from build123d import *

# Parameters (mm, degrees)
SKETCH1_W           = 55
SKETCH1_H           = 36
SKETCH1_R           = 2
BOSS_EXTRUDE1_DEPTH = 10
SKETCH2_W           = 7
SKETCH2_H           = 20
SKETCH2_H_2         = 17.5
BOSS_EXTRUDE2_DEPTH = 21
SKETCH3_R           = 1.25
CUT_EXTRUDE1_DEPTH  = 10
CUT_EXTRUDE2_DEPTH  = 5.5
LPATTERN1_COUNT     = 2
LPATTERN1_PITCH     = 28
FILLET1_R           = 1


with BuildPart() as part:
    # Sketch1 → Boss-Extrude1 (new body)
    with BuildSketch(Plane.XY):
        with Locations((27.5, -18)):
            Rectangle(SKETCH1_W, SKETCH1_H)
        with Locations((13.5, -4.5)):
            Circle(SKETCH1_R, mode=Mode.SUBTRACT)
        with Locations((41.5, -4.5)):
            Circle(SKETCH1_R, mode=Mode.SUBTRACT)
    extrude(amount=BOSS_EXTRUDE1_DEPTH)

    # Sketch2 → Boss-Extrude2 (add)
    with BuildSketch(Plane.XZ.offset(36)):
        with Locations((3.5, 20)):
            Rectangle(SKETCH2_W, SKETCH2_H)
        with Locations((51.5, 18.75)):
            Rectangle(SKETCH2_W, SKETCH2_H_2)
    extrude(amount=-BOSS_EXTRUDE2_DEPTH)

    # Sketch3 → Cut-Extrude1 (cut)
    with BuildSketch(Plane(origin=(0, -15, 0), x_dir=(1, 0, 0), z_dir=(0, 1, 0))):
        with Locations(Location((3.5, -15, 0), (0, 0, 270))):
            Circle(SKETCH3_R)
        with Locations(Location((51.5, -15, 0), (0, 0, 270))):
            Circle(SKETCH3_R)
        with Locations(Location((51.5, -25, 0), (0, 0, 270))):
            Circle(SKETCH3_R)
        with Locations(Location((3.5, -25, 0), (0, 0, 270))):
            Circle(SKETCH3_R)
    extrude(amount=-CUT_EXTRUDE1_DEPTH, mode=Mode.SUBTRACT)

    # Sketch4 → Cut-Extrude2 (cut)
    with BuildSketch(Plane.XY.offset(10)):
        Polygon((11.91228676, -1.75), (10.324573519, -4.5), (11.91228676, -7.25), (15.08771324, -7.25), (16.675426481, -4.5), (15.08771324, -1.75), align=None)
    cut_extrude2 = extrude(amount=-CUT_EXTRUDE2_DEPTH, mode=Mode.SUBTRACT)

    # LPattern1: Cut-Extrude2 ×2
    with Locations(*[(i * LPATTERN1_PITCH, 0, 0) for i in range(1, LPATTERN1_COUNT)]):
        add(cut_extrude2, mode=Mode.SUBTRACT)

    # Fillet1
    fillet1_edges = [part.edges().sort_by_distance(p)[0] for p in [
        (0, -25.5, 30),
        (7, -25.5, 30),
        (7, -25.5, 10),
        (55, -25.5, 27.5),
        (48, -25.5, 10),
        (48, -25.5, 27.5),
    ]]
    fillet(fillet1_edges, radius=FILLET1_R)


solid = part.part
Work out the finished part from the listing and answer in its coordinate system (mm). A direction names the side the tool comes from. Give positions to 0.01 mm unless a question says otherwise; leave off trailing zeros. Loops run counter-clockwise (first coordinate to the right, second up) from the corner with the lowest first, then second, coordinate; pieces in that order, holes last. Notation, with made-up numbers: (30.5, 54) - (42.5, 54) arc R21 cw to (42.5, 84) - close; hole circle Ø4 at (78, 18). An arc over 180 degrees is marked (long way). Answer in a Markdown table with one row per item.
(1) Section C-C (z = 12.75) is taken. Give the vertices of the cut face in (x, y), and give its area (3 significant figures).
Results list:
| item | result |
|---|---|
| outline | (0, -36) - (7, -36) - (7, -15) - (0, -15) - close; (48, -36) - (55, -36) - (55, -15) - (48, -15) - close |
| area | 294 mm² |
(2) Section A-A (x = 13.5) is taken. Give the vertices of the cut face in (y, z), and give its area (3 significant figures).
Results list:
| item | result |
|---|---|
| outline | (-36, 0) - (-6.5, 0) - (-6.5, 4.5) - (-7.25, 4.5) - (-7.25, 10) - (-36, 10) - close; (-2.5, 0) - (0, 0) - (0, 10) - (-1.75, 10) - (-1.75, 4.5) - (-2.5, 4.5) - close |
| area | 312 mm² |
(3) Section B-B (y = -19) is taken. Give the vertices of the cut face in (x, z).
Results list:
| item | result |
|---|---|
| outline | (0, 0) - (55, 0) - (55, 26.5) arc R1 ccw to (54, 27.5) - (49, 27.5) arc R1 ccw to (48, 26.5) - (48, 11) arc R1 cw to (47, 10) - (8, 10) arc R1 cw to (7, 11) - (7, 29) arc R1 ccw to (6, 30) - (1, 30) arc R1 ccw to (0, 29) - close; hole circle Ø2.5 at (3.5, 15); hole circle Ø2.5 at (3.5, 25); hole circle Ø2.5 at (51.5, 15); hole circle Ø2.5 at (51.5, 25) |
(4) For a pull along X with two mould halves and no side action, classify faces 6 (the face through (2.74, -19.93, 14.01)), 7 (the face through (27, -36, 9)) as pulls with the +X half, pulls with the -X half, needs draft (parallel to the pull), parting line crosses it, or undercut.
Results list:
| item | result |
|---|---|
| face 6 | undercut |
| face 7 | needs draft |
(5) Consider L1, parallel to X at y = -19, z = 15; L2, parallel to X at y = -4.5, z = 2.3; L3, parallel to Y at x = 14, z = 9. Determine where each line is inside the solid, lowest interval first. Write a range as [from, to].
Results list:
| item | result |
|---|---|
| L1 | x = [0, 2.25], [4.75, 7], [48, 50.25], [52.75, 55] |
| L2 | x = [0, 11.5], [15.5, 39.5], [43.5, 55] |
| L3 | y = [-36, -7.25], [-1.75, 0] |
(6) A tool of negligible diameter and unlimited length cuts with its end or side. For faces 1 (the face through (11.9, -5.7, 2.2)), 2 (the face through (52.74, -19.93, 24.84)), 3 (the face through (42, -1.75, 7)), 4 (the face through (7, -26, 20)), 5 (the face through (3, -26, 30)), from which of +Z, -Z, +X, -X, +Y, -Y can it reach the whole face along a straight path? Write none if from no direction.
Results list:
| item | result |
|---|---|
| face 1 | +Z, -Z |
| face 2 | +Y |
| face 3 | +Z |
| face 4 | +Z, +Y, -Y |
| face 5 | +Z, +X, -X, +Y, -Y |
(7) Flat-ended cylindrical pins translate along their axes: pin 1 Ø3 at (x, z) = (43, 13) entering from -Y; pin 2 Ø3 at (x, z) = (51.5, 15) entering from +Y; pin 3 Ø18 at (x, y) = (29.5, -15.5) entering from +Z; pin 4 Ø1.5 at (x, z) = (51.5, 25) entering from +Y. Find the tip coordinate at first contact, or state that the pin passes through.
Results list:
| item | result |
|---|---|
| pin 1 | passes through |
| pin 2 | stops at y = -15 |
| pin 3 | stops at z = 10 |
| pin 4 | stops at y = -25 |
(8) Section D-D (y = -31.5) is taken. Give the vertices of the cut face in (x, z).
Results list:
| item | result |
|---|---|
| outline | (0, 0) - (55, 0) - (55, 26.5) arc R1 ccw to (54, 27.5) - (49, 27.5) arc R1 ccw to (48, 26.5) - (48, 11) arc R1 cw to (47, 10) - (8, 10) arc R1 cw to (7, 11) - (7, 29) arc R1 ccw to (6, 30) - (1, 30) arc R1 ccw to (0, 29) - close |
